The listing builds one solid part. Answer for the finished solid, in the listing's coordinates (mm). Face numbers are marked on the shaded views. A direction names the side the tool comes from. Give positions to 0.01 mm unless a question says otherwise; leave off trailing zeros. Write each loop counter-clockwise with the first axis right and the second up, starting at its lowest first coordinate (ties: lowest second). Pieces come first, ordered by that corner, then holes.
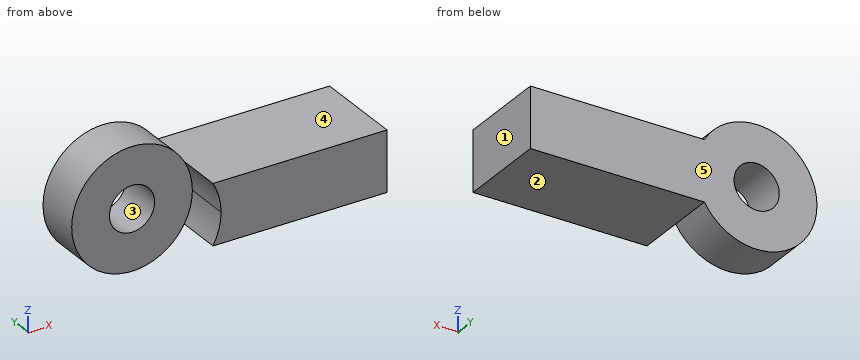
```python
from build123d import *

# Parameters (mm, degrees)
F0_R     = 7.5
F1_DEPTH = 15
F2_DEPTH = 30


with BuildPart() as f1:
    # F0 (on Front) → F1 (new body)
    with BuildSketch(Plane.XZ):
        with BuildLine():
            ThreePointArc((-2.679492, -10), (-0.681483, -5.176381), (0, 0))
            ThreePointArc((0, 0), (-0.681483, 5.176381), (-2.679492, 10))
            ThreePointArc((-2.679492, 10), (-40, 0), (-2.679492, -10))
        make_face()
        with Locations((-20, 0)):
            Circle(F0_R, mode=Mode.SUBTRACT)
    extrude(amount=F1_DEPTH)

    # F0 (on Front) → F2 (join)
    with BuildSketch(Plane.XZ):
        with BuildLine():
            ThreePointArc((-2.679492, 10), (-0.681483, 5.176381), (0, 0))
            ThreePointArc((0, 0), (-0.681483, -5.176381), (-2.679492, -10))
            Line((-2.679492, -10), (55, -10))
            Line((55, -10), (55, 10))
            Line((55, 10), (-2.679492, 10))
        make_face()
    extrude(amount=F2_DEPTH)


solid = f1.part
```
Item 1: A cutting plane is placed at D-D, the plane y = -23.5. Give the vertices of the cut face in (x, z).
Conclusion:
outline: (-2.68, -10) - (55, -10) - (55, 10) - (-2.68, 10) arc R20 cw to (0, 0) arc R20 cw to start
Item 2: A cutting plane is placed at A-A, the plane x = -20. Give the vertices of the cut face in (y, z).
Conclusion:
outline: (-15, -20) - (0, -20) - (0, -7.5) - (-15, -7.5) - close; (-15, 7.5) - (0, 7.5) - (0, 20) - (-15, 20) - close
Item 3: Determine the mould class of the marked faces 1, 2 and 3 for opening direction X: pulls with the +X half, pulls with the -X half, needs draft (parallel to the pull), parting line crosses it, or undercut.
Conclusion:
face 1: pulls with the +X half
face 2: needs draft
face 3: undercut
Item 4: Each of these flat-tipped pins is pushed along its axis until it touches: P1, Ø6, axis at x = -5, y = -26, coming from the -Z side; P2, Ø17, axis at x = -20, z = 0, coming from the -Y side; P3, Ø3, axis at x = 3, y = -3, coming from the +Z side. Where does it stop, or does it pass through?
Conclusion:
P1: stops at z = -10
P2: stops at y = -15
P3: stops at z = 10
Item 5: A cutting plane is placed at B-B, the plane y = -13.5. Give the vertices of the cut face in (x, z), plus the area to 3 significant figures.
Conclusion:
outline: (-2.68, -10) - (55, -10) - (55, 10) - (-2.68, 10) arc R20 ccw (long way) to start; hole circle Ø15 at (-20, 0)
area: 2,200 mm2
Item 6: Consider probe 1 along Z at (x, y) = (-20, -8.25); probe 2 along Z at (x, y) = (50.5, -19.5); probe 3 along Y at (x, z) = (-12, -8.5). Determine where each line is inside the solid, lowest interval first.
Conclusion:
probe 1: z = -20 to -7.5, 7.5 to 20
probe 2: z = -10 to 10
probe 3: y = -15 to 0
Item 7: A cutting plane is placed at C-C, the plane z = 2. Give the vertices of the cut face in (x, y).
Conclusion:
outline: (-39.9, -15) - (-27.23, -15) - (-27.23, 0) - (-39.9, 0) - close; (-12.77, -15) - (-0.1, -15) - (-0.1, -30) - (55, -30) - (55, 0) - (-12.77, 0) - close
Item 8: Which of the six approach directions +Z, -Z, +X, -X, +Y, -Y give full straight-line access (tool end or side, diameter ignored) to the marked faces 4 and 5?
Conclusion:
face 4: +Z, +X, +Y, -Y
face 5: +Z, -Z, +X, -X, +Y
